Source: CAD feature listing. Evaluate the final solid. Frame: model axes, mm. Face numbers are marked on the shaded views. Round coordinates to 2 decimals unless told otherwise and drop trailing zeros. Loops run counter-clockwise (first coordinate to the right, second up) from the corner with the lowest first, then second, coordinate; pieces in that order, holes last. Notation, with made-up numbers: M 14.25,5 L 45.25,5 A15 cw 45.25,17 Z; hole C -37.5,6.25 d6. An arc over 180 degrees is marked long. Answer as a JSON object with one key per item and string values.
from build123d import *

# Parameters (mm, degrees)
F0_R     = 32
F0_R_2   = 7.5
F1_DEPTH = 3
F2_R     = 27
F2_R_2   = 11
F3_DEPTH = 7
F4_SIZE  = 0.5


with BuildPart() as f1:
    # F0 (on Top) → F1 (new body)
    with BuildSketch(Plane.XY):
        Circle(F0_R)
        Circle(F0_R_2, mode=Mode.SUBTRACT)
    extrude(amount=F1_DEPTH)

    # F2 (on face) → F3 (join)
    with BuildSketch(Plane.XY.offset(3)):
        Circle(F2_R)
        Circle(F2_R_2, mode=Mode.SUBTRACT)
    extrude(amount=F3_DEPTH)

    # F4
    f4_edges = [f1.edges().sort_by_distance(p)[0] for p in [
        (-27, 0, 10),
        (-32, 0, 3),
        (-11, 0, 10),
        (-32, 0, 0),
        (-7.5, 0, 0),
    ]]
    chamfer(f4_edges, length=F4_SIZE)


solid = f1.part
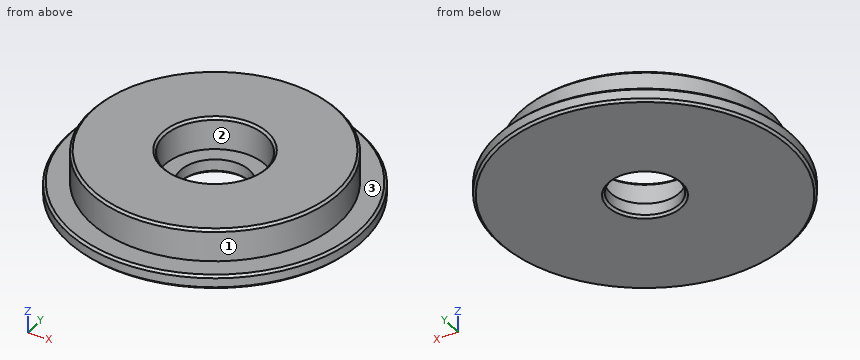
Item 1: Pull-direction query (Y, two-part tool) for the marked faces 1, 2 and 3; classes: pulls with the +Y half, pulls with the -Y half, needs draft (parallel to the pull), parting line crosses it, or undercut.
Answer sheet:
{"face 1": "parting line crosses it", "face 2": "undercut", "face 3": "needs draft"}
Item 2: Contact query for flat-ended pins moving along their axis: pin 1 Ø12 at (x, y) = (0, 0) entering from -Z; pin 2 Ø6.5 at (x, y) = (2, -4.5) entering from +Z; pin 3 Ø1.5 at (x, y) = (20, 20.5) entering from -Z; pin 4 Ø1 at (x, z) = (-20, 8) entering from -Y. Output: stop coordinate, or through.
Answer sheet:
{"pin 1": "passes through", "pin 2": "stops at z = 3", "pin 3": "stops at z = 0", "pin 4": "stops at y = -18.67"}
Item 3: Line query: probe 1 along Y at (x, z) = (0, 1.55); probe 2 along X at (y, z) = (-0.5, 6.5); probe 3 along Z at (x, y) = (23, 21). Output: solid intervals per line, ascending. Write a range as from..to.
Answer sheet:
{"probe 1": "y = -32..-7.5, 7.5..32", "probe 2": "x = -27..-10.99, 10.99..27", "probe 3": "z = 0..3"}
Item 4: Section C-C on z = 4.25. Return the cut outline in (x, y).
Answer sheet:
{"outline": "C 0,0 d54; hole C 0,0 d22"}
Item 5: Section A-A on x = 0. Return the cut outline in (y, z).
Answer sheet:
{"outline": "M -32,0.5 L -31.5,0 L -8,0 L -7.5,0.5 L -7.5,3 L -11,3 L -11,9.5 L -11.5,10 L -26.5,10 L -27,9.5 L -27,3 L -31.5,3 L -32,2.5 Z; M 7.5,0.5 L 8,0 L 31.5,0 L 32,0.5 L 32,2.5 L 31.5,3 L 27,3 L 27,9.5 L 26.5,10 L 11.5,10 L 11,9.5 L 11,3 L 7.5,3 Z"}
